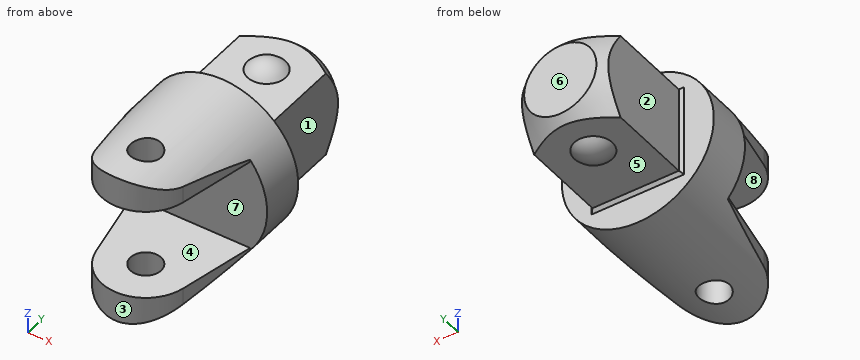
```python
from build123d import *

# Parameters (mm, degrees)
SKETCH1_R           = 12
BOSS_EXTRUDE1_DEPTH = 33.53
CUT_EXTRUDE1_DEPTH  = 19.6
CHAMFER1_SIZE       = 0.4
SKETCH3_R           = 9.375
CUT_EXTRUDE2_DEPTH  = 3.4
CUT_EXTRUDE2_DRAFT  = -35
SKETCH4_W           = 24
SKETCH4_H           = 14.42225279
CUT_EXTRUDE3_DEPTH  = 17.4
SKETCH5_R           = 2.415
CUT_EXTRUDE4_DEPTH  = 33.7
CUT_EXTRUDE5_START  = -9
SKETCH6_R           = 12
CUT_EXTRUDE5_DEPTH  = 9
BOSS_EXTRUDE2_START = -7.13
SKETCH7_R           = 12
BOSS_EXTRUDE2_DEPTH = 7.13
SKETCH8_W           = 13.62
SKETCH8_H           = 13.62
BOSS_EXTRUDE3_DEPTH = 17.8
CHAMFER2_SIZE       = 0.5


with BuildPart() as part:
    # Sketch1 → Boss-Extrude1 (new body)
    with BuildSketch(Plane(origin=(0, 0, 0), x_dir=(1, 0, 0), z_dir=(0, 1, 0))):
        with Locations(Location((0, 0, 0), (0, 0, 270))):
            Circle(SKETCH1_R)
    extrude(amount=BOSS_EXTRUDE1_DEPTH)

    # Sketch2 → Cut-Extrude1 (cut)
    with BuildSketch(Plane(origin=(0, 33.53, 0), x_dir=(1, 0, 0), z_dir=(0, 1, 0))):
        with BuildLine():
            Line((-6.5, 6.5), (-2.5, 6.5))
            ThreePointArc((-2.5, 6.5), (0, 7.211126395), (2.5, 6.5))
            Line((2.5, 6.5), (6.5, 6.5))
            Line((6.5, 6.5), (6.5, 2.5))
            ThreePointArc((6.5, 2.5), (7.211126395, 0), (6.5, -2.5))
            Line((6.5, -2.5), (6.5, -6.5))
            Line((6.5, -6.5), (2.5, -6.5))
            ThreePointArc((2.5, -6.5), (0, -7.211126395), (-2.5, -6.5))
            Line((-2.5, -6.5), (-6.5, -6.5))
            Line((-6.5, -6.5), (-6.5, -2.5))
            ThreePointArc((-6.5, -2.5), (-7.211126395, 0), (-6.5, 2.5))
            Line((-6.5, 2.5), (-6.5, 6.5))
        make_face()
    extrude(amount=-CUT_EXTRUDE1_DEPTH, mode=Mode.SUBTRACT)

    # Chamfer1
    chamfer1_edges = [part.edges().sort_by_distance(p)[0] for p in [
        (-6.5, 23.73, -6.5),
        (6.5, 23.73, -6.5),
        (6.5, 23.73, 6.5),
        (-6.5, 23.73, 6.5),
    ]]
    chamfer(chamfer1_edges, length=CHAMFER1_SIZE)


with BuildPart() as cut_extrude2_tool:
    # Sketch3 → Cut-Extrude2 (with draft: the straight prism first)
    with BuildSketch(Plane(origin=(0, 33.53, 0), x_dir=(1, 0, 0), z_dir=(0, 1, 0))):
        Circle(SKETCH3_R)
    extrude(amount=-CUT_EXTRUDE2_DEPTH)
    # Cut-Extrude2: the draft: its side faces are tilted about the plane it starts from
    cut_extrude2_sides = [cut_extrude2_tool.faces().sort_by_distance(p)[0] for p in [
        (-9.375, 31.83, 0),
    ]]
    draft(cut_extrude2_sides, Plane(origin=(0, 33.53, 0), x_dir=(1, 0, 0), z_dir=(0, 1, 0)), CUT_EXTRUDE2_DRAFT)


with BuildPart() as part_1:
    add(part.part)

    # Cut-Extrude2: cut by cut_extrude2_tool
    add(cut_extrude2_tool.part, mode=Mode.SUBTRACT)

    # Sketch4 → Cut-Extrude3 (cut)
    with BuildSketch(Plane.XZ):
        Rectangle(SKETCH4_W, SKETCH4_H)
    extrude(amount=-CUT_EXTRUDE3_DEPTH, mode=Mode.SUBTRACT)

    # Sketch5 → Cut-Extrude4 (cut, symmetric)
    with BuildSketch(Plane.XY):
        with Locations(Location((0, 7, 0), (0, 0, 90))):
            Circle(SKETCH5_R)
        with BuildLine():
            ThreePointArc((-6.854820161, 5.581747356), (0, 0), (6.854820161, 5.581747356))
            Line((6.854820161, 5.581747356), (9.3, 17.4))
            Line((9.3, 17.4), (12, 17.4))
            Line((12, 17.4), (12, -3.192277431))
            Line((12, -3.192277431), (-12, -3.192277431))
            Line((-12, -3.192277431), (-12, 17.4))
            Line((-12, 17.4), (-9.3, 17.4))
            Line((-9.3, 17.4), (-6.854820161, 5.581747356))
        make_face()
    extrude(amount=CUT_EXTRUDE4_DEPTH, both=True, mode=Mode.SUBTRACT)

    # Sketch6 → Cut-Extrude5 (cut)
    with BuildSketch(Plane(origin=(0, 33.53, 0), x_dir=(1, 0, 0), z_dir=(0, 1, 0)).offset(CUT_EXTRUDE5_START)):
        with Locations(Location((0, 0, 0), (0, 0, 55.16360803))):
            Circle(SKETCH6_R)
    extrude(amount=CUT_EXTRUDE5_DEPTH, mode=Mode.SUBTRACT)

    # Sketch7 → Boss-Extrude2 (add)
    with BuildSketch(Plane(origin=(0, 24.53, 0), x_dir=(1, 0, 0), z_dir=(0, 1, 0)).offset(BOSS_EXTRUDE2_START)):
        with Locations(Location((0, 0, 0), (0, 0, 55.16360803))):
            Circle(SKETCH7_R)
    extrude(amount=BOSS_EXTRUDE2_DEPTH)

    # Sketch8 → Boss-Extrude3 (add)
    with BuildSketch(Plane(origin=(0, 24.53, 0), x_dir=(1, 0, 0), z_dir=(0, 1, 0))):
        Rectangle(SKETCH8_W, SKETCH8_H)
    extrude(amount=BOSS_EXTRUDE3_DEPTH)

    # Sketch9 → Cut-Revolve1 (revolve, cut)
    with BuildSketch(Plane.XY, mode=Mode.PRIVATE) as cut_revolve1_sk:
        Polygon((5.7, 42.33), (13.111265215, 42.33), (13.111265215, 34.918734785), align=None)
    revolve(cut_revolve1_sk.sketch.rotate(Axis((0, 44.4465, 0), (0, -1, 0)), 304.83639197), axis=Axis((0, 44.4465, 0), (0, -1, 0)), mode=Mode.SUBTRACT)

    # Chamfer2
    chamfer2_edges = [part_1.edges().sort_by_distance(p)[0] for p in [
        (6.81, 24.53, 0),
        (0, 24.53, -6.81),
        (-6.81, 24.53, 0),
        (0, 24.53, 6.81),
    ]]
    chamfer(chamfer2_edges, length=CHAMFER2_SIZE)

    # Sketch10 → Revolve1 (revolve)
    with BuildSketch(Plane(origin=(0, 0, 0), x_dir=(0, 0, -1), z_dir=(1, 0, 0))):
        with BuildLine():
            Line((6.81, 34.73), (6.81, 31.73))
            ThreePointArc((6.81, 31.73), (7.806952033, 33.085121585), (8.16, 34.73))
            Line((8.16, 34.73), (6.81, 34.73))
        make_face()
    revolve1 = revolve(axis=Axis((0, 34.73, -6.81), (0, 0, -1)))

    # Mirror1: Revolve1 across plane
    add(revolve1.mirror(Plane.XY))


solid = part_1.part
```
Design review of the part built by this model. Coordinates are the model's own, in mm. Face numbers are marked on the shaded views. A direction names the side the tool comes from. Coordinates: 2 decimals unless noted, no trailing zeros. Loops run counter-clockwise (first coordinate to the right, second up) from the corner with the lowest first, then second, coordinate; pieces in that order, holes last.
Q1. We need section A-A on x = 0. State the section outline as (y, z) points (3 decimals), and give its area (3 significant figures).
Reported:
outline: (0, -12) - (4.585, -12) - (4.585, -7.211) - (0, -7.211) - close; (0, 7.211) - (4.585, 7.211) - (4.585, 12) - (0, 12) - close; (9.415, -12) - (24.53, -12) - (24.53, -7.31) - (25.03, -6.81) - (31.73, -6.81) arc R4.008 ccw to (37.73, -6.81) - (41.22, -6.81) - (42.33, -5.7) - (42.33, 5.7) - (41.22, 6.81) - (37.73, 6.81) arc R4.008 ccw to (31.73, 6.81) - (25.03, 6.81) - (24.53, 7.31) - (24.53, 12) - (9.415, 12) - (9.415, 7.211) - (17.4, 7.211) - (17.4, -7.211) - (9.415, -7.211) - close
area: 544 mm2
Q2. The part is to be moulded in two halves that separate along Z. For the marked faces 5, 6, 7 and 8, say which applies: +Z half, -Z half, draft (parallel to the pull), parting line (faces both ways), or undercut.
Reported:
face 5: -Z half
face 6: draft
face 7: undercut
face 8: undercut
Q3. Tool access review of the marked faces 1, 2, 3 and 4: name each direction out of +Z, -Z, +X, -X, +Y, -Y from which nothing blocks a thin tool from reaching the whole face with its end or side.
Reported:
face 1: +Z, -Z, +X, +Y
face 2: +Z, -Z, -X, +Y
face 3: +Z, -Z, -Y
face 4: +X, -X, -Y
Q4. For pin 1 (12 mm diameter, centred on x = 4.5, z = -2.5, fed in from -Y); pin 2 (1.5 mm diameter, centred on x = -3, z = -4, fed in from -Y); pin 3 (1 mm diameter, centred on x = -2.5, z = -9, fed in from +Y), all flat-tipped, find the tip position at first contact; note any pin that passes through.
Reported:
pin 1: stops at y = 0.04
pin 2: stops at y = 17.4
pin 3: stops at y = 24.53
Q5. We need section B-B on y = 16. State the section outline as (x, z) points, and give its area (3 significant figures).
Reported:
outline: (-9.01, -7.93) arc R12 ccw to (9.01, -7.93) - (9.01, -7.21) - (-9.01, -7.21) - close; (-9.01, 7.21) - (9.01, 7.21) - (9.01, 7.93) arc R12 ccw to (-9.01, 7.93) - close
area: 128 mm2
Q6. To check wall thickness, follow line 1 (Y direction, x = 0, z = 9.75) (3 decimals); line 2 (Z direction, x = -5.75, y = 38); line 3 (Z direction, x = 6.75, y = 15.5). State the ranges of each line that lie inside material, in increasing order.
Reported:
line 1: y = 0 to 4.585, 9.415 to 24.53
line 2: z = -6.81 to 6.81
line 3: z = -9.92 to -7.21, 7.21 to 9.92
Q7. We need section C-C on z = 0. State the section outline as (x, y) points.
Reported:
outline: (-12, 17.4) - (12, 17.4) - (12, 24.53) - (7.31, 24.53) - (6.81, 25.03) - (6.81, 41.22) - (5.7, 42.33) - (-5.7, 42.33) - (-6.81, 41.22) - (-6.81, 25.03) - (-7.31, 24.53) - (-12, 24.53) - close
Q8. We need section D-D on y = 7. State the section outline as (x, z) points (3 decimals).
Reported:
outline: (-7.148, -9.639) arc R12 ccw to (-2.415, -11.754) - (-2.415, -7.211) - (-7.148, -7.211) - close; (-7.148, 7.211) - (-2.415, 7.211) - (-2.415, 11.754) arc R12 ccw to (-7.148, 9.639) - close; (2.415, -11.754) arc R12 ccw to (7.148, -9.639) - (7.148, -7.211) - (2.415, -7.211) - close; (2.415, 7.211) - (7.148, 7.211) - (7.148, 9.639) arc R12 ccw to (2.415, 11.754) - close
